Design review of the part built by this model. Coordinates are the model's own, in mm. A direction names the side the tool comes from. Give positions to 0.01 mm unless a question says otherwise; leave off trailing zeros. Loops run counter-clockwise (first coordinate to the right, second up) from the corner with the lowest first, then second, coordinate; pieces in that order, holes last. Notation, with made-up numbers: (67.25, 56) -> (76.25, 56) arc R10 cw to (76.25, 60) -> close; hole circle Ø3 at (74.25, 85.25). An arc over 180 degrees is marked (long way). Use a Markdown table: item, result. Add a question column.
1. For faces 5 (the flat face through (0, -40.8, 6)), 6 (the flat face through (-11.45, 45, 6)), 7 (the flat face through (0, -43.8, 6)), 8 (the flat face through (-14, 39, 2)), list the 3-axis set-ups (+Z, -Z, +X, -X, +Y, -Y) from which the entire face can be reached by the end or side of a thin tool; tool diameter is ignored.
2. Add section C-C (z = 6.5). Count the separate pieces of the cut face and the enclosed holes in it, and give its area (3 significant figures).
3. Add section A-A (y = -12.5). State the section outline as (x, z) points.
4. Add section D-D (x = 13.5). State the section outline as (y, z) points.
5. Draft analysis for pull direction X (two halves, no side actions). For faces 1 (the flat face through (21.45, 1, 6)), 2 (the flat face through (7.5, 39, 6)), 3 (the cylindrical face through (-20.85, 46.13, 6.08)), 4 (the flat face through (-16, -46.7, 6)), state which applies: pulls with the +X half, pulls with the -X half, needs draft (parallel to the pull), parting line crosses it, or undercut.
6. To check wall thickness, follow line 1 (X direction, y = 38.8, z = 5.5); line 2 (Y direction, x = -6, z = 6); line 3 (Y direction, x = 13, z = 3.5). State the ranges of each line that lie inside material, in increasing order.
7. Add section B-B (x = -16.45). State the section outline as (y, z) points.
8. For pin 1 Ø1.5 at (x, z) = (-8, 3) entering from -Y; pin 2 Ø0.9 at (y, z) = (45.5, 8.5) entering from +X; pin 3 Ø0.9 at (y, z) = (-46, 7) entering from +X, all flat-tipped, find the tip position at first contact; note any pin that passes through.
Autodesk Inventor part; units mm, degrees
ref_plane "YZ Plane" through (0, 0, 0) normal (1, 0, 0) x (0, 1, 0)
ref_plane "XZ Plane" through (0, 0, 0) normal (0, 1, 0) x (-1, 0, 0)
ref_plane "XY Plane" through (0, 0, 0) normal (0, 0, 1) x (1, 0, 0)
sketch "Эскиз1" plane through (0, 0, 0) normal (0, 0, 1) x (1, 0, 0)
  line L0 (-18.25, -37.6) -> (18.25, -37.6)
  line L1 (18.25, -37.6) -> (18.25, 37.6)
  line L2 (18.25, 37.6) -> (-18.25, 37.6)
  line L3 (-18.25, 37.6) -> (-18.25, -37.6)
  line L4 (-18.25, 0) -> (18.25, 0) construction
  line L5 (0, 37.6) -> (0, -37.6) construction
  line L6 (-18.45, -37.8) -> (18.45, -37.8)
  line L7 (18.45, -37.8) -> (18.45, 37.8)
  line L8 (18.45, 37.8) -> (-18.45, 37.8)
  line L9 (-18.45, 37.8) -> (-18.45, -37.8)
  line L10 (-7.5, -37.8) -> (7.5, -37.8)
  line L11 (7.5, -37.8) -> (7.5, -40.8)
  line L12 (7.5, -40.8) -> (-7.5, -40.8)
  line L13 (-7.5, -40.8) -> (-7.5, -37.8)
  line L14 (-18.45, -37.8) -> (-18.45, -43.8)
  line L15 (-18.45, -43.8) -> (18.45, -43.8)
  line L16 (18.45, -43.8) -> (18.45, -37.8)
  line L17 (-18.45, 43.8) -> (18.45, 43.8)
  line L18 (-18.45, 37.8) -> (-18.45, 43.8)
  line L19 (18.45, 43.8) -> (18.45, 37.8)
  line L20 (-18.45, -43.8) -> (-21.45, -43.8)
  line L21 (-21.45, -43.8) -> (-21.45, 43.8)
  line L22 (-21.45, 43.8) -> (-18.45, 43.8)
  line L23 (-18.45, 43.8) -> (-18.45, -43.8)
  line L24 (21.45, 43.8) -> (18.45, 43.8)
  line L25 (18.45, 37.8) -> (18.45, 43.8)
  line L26 (18.45, 43.8) -> (18.45, -43.8)
  line L27 (21.45, -43.8) -> (21.45, 43.8)
  line L28 (-7.5, 40.8) -> (-7.5, 37.8)
  line L29 (7.5, 40.8) -> (-7.5, 40.8)
  line L30 (7.5, 37.8) -> (7.5, 40.8)
  line L31 (-21.45, -43.8) -> (-11.45, -43.8)
  line L32 (18.45, -43.8) -> (21.45, -43.8)
  line L33 (21.45, -43.8) -> (11.45, -43.8)
  line L34 (16.45, 46.7) -> (21.45, 46.7)
  line L35 (16.45, 46.7) -> (11.45, 46.7)
  line L36 (11.45, 46.7) -> (11.45, 43.8)
  line L37 (21.45, 46.7) -> (21.45, 43.8)
  line L38 (11.45, 43.8) -> (16.45, 43.8)
  line L39 (-11.45, 46.7) -> (-11.45, 43.8)
  line L40 (-16.45, 46.7) -> (-11.45, 46.7)
  line L41 (-16.45, 46.7) -> (-21.45, 46.7)
  line L42 (-21.45, 46.7) -> (-21.45, 43.8)
  line L43 (-16.45, -46.7) -> (-21.45, -46.7)
  line L44 (-21.45, -46.7) -> (-21.45, -43.8)
  line L45 (-16.45, -46.7) -> (-11.45, -46.7)
  line L46 (-11.45, -46.7) -> (-11.45, -43.8)
  line L47 (11.45, -46.7) -> (11.45, -43.8)
  line L48 (16.45, -46.7) -> (11.45, -46.7)
  line L49 (16.45, -46.7) -> (21.45, -46.7)
  line L50 (21.45, -46.7) -> (21.45, -43.8)
  circle A0 centre (16.45, -43.8) radius 1.5
  circle A1 centre (-16.45, -43.8) radius 1.5
  circle A2 centre (16.45, 43.8) radius 1.5
  circle A3 centre (-16.45, 43.8) radius 1.5
  line L51 (0, 0) -> (-14.3, 0) construction
  line L52 (-14.3, 0) -> (-14.3, 38.8) construction
  line L53 (-14.3, 38.8) -> (0, 38.8) construction
  line L54 (0, 38.8) -> (0, 0) construction
  circle A4 centre (-14.3, 38.8) radius 1.25
  point P0 (-1.9914, -32.8601)
  point P1 (0, -37.8)
  point P2 (-15.05, 37.8)
  point P3 (-13.55, 37.8)
  dimension "d0" = 36.5
  dimension "d1" = 75.2
  dimension "d2" = 36.9
  dimension "d3" = 75.6
  dimension "d4" = 15
  dimension "d5" = 3
  dimension "d6" = 6
  dimension "d7" = 3
  dimension "d8" = 5
  dimension "d10" = 3
  dimension "d11" = 3
  dimension "d12" = 3
  dimension "d13" = 3
  dimension "d19" = 14.3
  dimension "d20" = 38.8
  dimension "d21" = 2.5
extrude "Выдавливание1" add sketch "Эскиз1" along normal blind 12 contours A4 L8 | L8 L18 L17 A3 A2 L19 L30 L29 L28 A4 | L9 L14 L20 L21 L22 L18 | L6 L13 L12 L11 L16 L15 A0 A1 L14 | L22 L42 L41 L40 L39 L17 A3 | L15 A1 L46 L45 L43 L44 L20 | L19 L24 L27 L32 L16 L7 | L17 A2 L36 L35 L34 L37 L24 | L32 L50 L49 L48 L47 L15 A0
fillet "Сопряжение1" radius 2 4 edges at (-21.45, 46.7, 6) (21.45, 46.7, 6) (-21.45, -46.7, 6) (21.45, -46.7, 6)
extrude "Выдавливание3" cut sketch "Эскиз1" against normal blind 10 from surface at 12 contours A4 L8
sketch "Эскиз2" plane through (-11.45, 43.8, 0) normal (0, 1, 0) x (1, 0, 0)
  line L0 (32.9, 0) -> (32.9, -12) construction
  line L1 (32.9, -6) -> (-10, -6) construction
  line L2 (-10, -12) -> (-10, 0) construction
  line L3 (3.95, -12) -> (18.95, -12) construction
  line L4 (11.45, -12) -> (11.45, 0) construction
  line L5 (32.9, -12) -> (30.9, -12) construction
  line L6 (32.9, -12) -> (11.45, -12) construction
  line L7 (11.45, -12) -> (11.45, -9.9) construction
  line L8 (11.45, -9.9) -> (32.9, -9.9) construction
  line L9 (32.9, -9.9) -> (32.9, -12) construction
  circle A0 centre (11.45, -9.9) radius 1.5
  dimension "d24" = 2.1
  dimension "d25" = 3
extrude "Выдавливание4" cut sketch "Эскиз2" against normal blind 3
properties part number "fast_akkum2"
Taken from the geometry:
| question | item | result |
|---|---|---|
| 1 | face 5 | +Z, -Z |
| 1 | face 6 | +Z, -Z, +Y |
| 1 | face 7 | +Z, -Z, -Y |
| 1 | face 8 | +Z |
| 2 | separate pieces | 1 |
| 2 | enclosed holes | 5 |
| 2 | area | 958 mm^2 |
| 3 | outline | (-21.45, 0) -> (-18.45, 0) -> (-18.45, 12) -> (-21.45, 12) -> close; (18.45, 0) -> (21.45, 0) -> (21.45, 12) -> (18.45, 12) -> close |
| 4 | outline | (-46.7, 0) -> (-37.8, 0) -> (-37.8, 12) -> (-46.7, 12) -> close; (37.8, 0) -> (46.7, 0) -> (46.7, 12) -> (37.8, 12) -> close |
| 5 | face 1 | pulls with the +X half |
| 5 | face 2 | undercut |
| 5 | face 3 | pulls with the -X half |
| 5 | face 4 | needs draft |
| 6 | line 1 | x = -21.45 to -15.55, -13.05 to -7.5, 7.5 to 21.45 |
| 6 | line 2 | y = -43.8 to -40.8, 40.8 to 43.8 |
| 6 | line 3 | y = -46.7 to -37.8, 37.8 to 46.7 |
| 7 | outline | (-46.7, 0) -> (-45.3, 0) -> (-45.3, 12) -> (-46.7, 12) -> close; (-42.3, 0) -> (-37.8, 0) -> (-37.8, 12) -> (-42.3, 12) -> close; (37.8, 0) -> (42.3, 0) -> (42.3, 12) -> (37.8, 12) -> close; (45.3, 0) -> (46.7, 0) -> (46.7, 12) -> (45.3, 12) -> close |
| 8 | pin 1 | stops at y = -43.8 |
| 8 | pin 2 | stops at x = 21.42 |
| 8 | pin 3 | stops at x = 21.26 |
